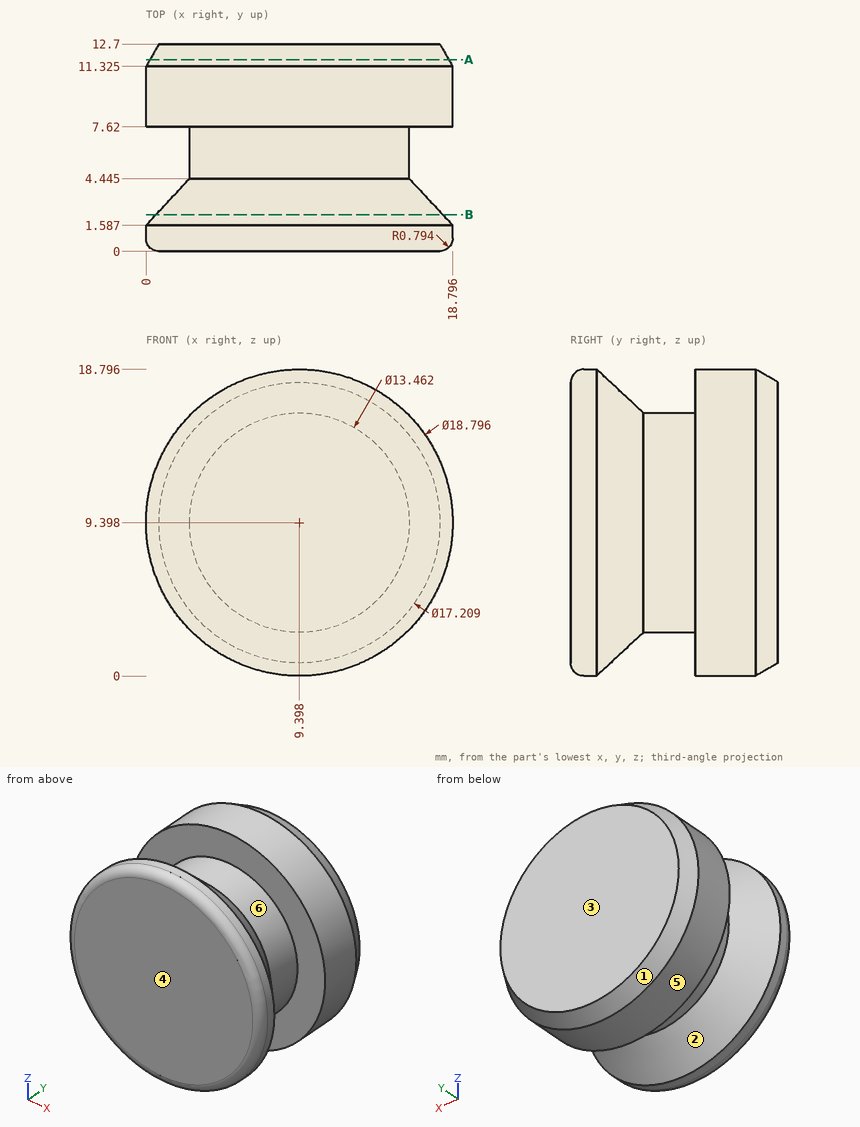
Source: three-view drawing plus pictorial views. Frame: mm from the lowest corner of the part. A direction names the side the tool comes from. Give positions to 0.01 mm unless a question says otherwise; leave off trailing zeros. Order: outer loops, then holes, each group sorted by start corner. A loop starts at its lowest first (then second) coordinate and runs counter-clockwise, first axis right, second up. Notation, with made-up numbers: (6.5, -27) -> (48.5, -27) arc R22 cw to (48.5, -12) -> close; hole circle Ø1 at (89.5, -24). An arc over 180 degrees is marked (long way). Use a Markdown table: item, result.
Q1. Section B-B (y = 2.25). Return the cut outline in (x, z), and give its area (3 significant figures).
A:
| item | result |
|---|---|
| outline | circle Ø17.56 at (9.4, 9.4) |
| area | 242 mm^2 |
Q2. Section A-A (y = 11.75). Return the cut outline in (x, z) (1 decimal).
A:
| item | result |
|---|---|
| outline | circle Ø18.3 at (9.4, 9.4) |
Q3. Pull-direction query (Y, two-part tool) for the marked faces 3, 4, 5 and 6; classes: +Y half, -Y half, draft (parallel to the pull), parting line (faces both ways), or undercut.
A:
| item | result |
|---|---|
| face 3 | +Y half |
| face 4 | -Y half |
| face 5 | draft |
| face 6 | undercut |
Q4. Access query for the marked faces 1 and 2. Directions: +Z, -Z, +X, -X, +Y, -Y. A direction counts if a zero-diameter tool reaches every point of the face in a straight line with its end or side. Return the directions, or none.
A:
| item | result |
|---|---|
| face 1 | +Y |
| face 2 | none |
Q5. First-contact query: P1, Ø6, axis at y = 5.5, z = 14.5, coming from the -X side (1 decimal); P2, Ø1.5, axis at x = 4.5, y = 6, coming from the +Z side; P3, Ø5, axis at y = 2.5, z = 2, coming from the +X side. Flat tips, straight axial feed; report the tip coordinate or a pass-through.
A:
| item | result |
|---|---|
| P1 | x = 0.5 |
| P2 | z = 14.7 |
| P3 | x = 17.31 |
Q6. Material intervals for line 1 (Z direction, x = 9.5, y = 1.5) (1 decimal); line 2 (Y direction, x = 1.25, z = 11); line 3 (Y direction, x = 17.25, z = 10.5), sorted ascending. Write a range as [from, to].
A:
| item | result |
|---|---|
| line 1 | [0, 18.8] |
| line 2 | [0, 2.76], [7.62, 12.7] |
| line 3 | [0, 3.16], [7.62, 12.7] |
